```python
from build123d import *

# Parameters (mm, degrees)
SKETCH2_W                  = 25.50248159
SKETCH2_H                  = 21.40954602
BOSS_EXTRUDE1_DEPTH        = 4
M2_5_CLEARANCE_HOLE1_D     = 2.7
M2_5_CLEARANCE_HOLE1_DEPTH = 6.65
M2_5_CLEARANCE_HOLE1_TIP   = 0.811161836
SKETCH6_R                  = 4.5
CUT_EXTRUDE1_DEPTH         = 18.12268399


with BuildPart() as part:
    # Sketch2 → Boss-Extrude1 (new body)
    with BuildSketch(Plane(origin=(0, 0, 0), x_dir=(0, 0, -1), z_dir=(1, 0, 0))):
        Rectangle(SKETCH2_W, SKETCH2_H)
    extrude(amount=BOSS_EXTRUDE1_DEPTH)

    # M2.5 Clearance Hole1
    with Locations(Plane.ZY):
        with Locations((0, 7), (-6.062177826, -3.5), (6.062177826, -3.5)):
            Hole(M2_5_CLEARANCE_HOLE1_D / 2, depth=M2_5_CLEARANCE_HOLE1_DEPTH)
            with Locations((0, 0, -(M2_5_CLEARANCE_HOLE1_DEPTH + M2_5_CLEARANCE_HOLE1_TIP / 2))):  # 118° drill point
                Cone(0, M2_5_CLEARANCE_HOLE1_D / 2, M2_5_CLEARANCE_HOLE1_TIP, mode=Mode.SUBTRACT)

    # Sketch6 → Cut-Extrude1 (cut, through all)
    with BuildSketch(Plane.ZY):
        Circle(SKETCH6_R)
    extrude(amount=-CUT_EXTRUDE1_DEPTH, mode=Mode.SUBTRACT)


solid = part.part
```
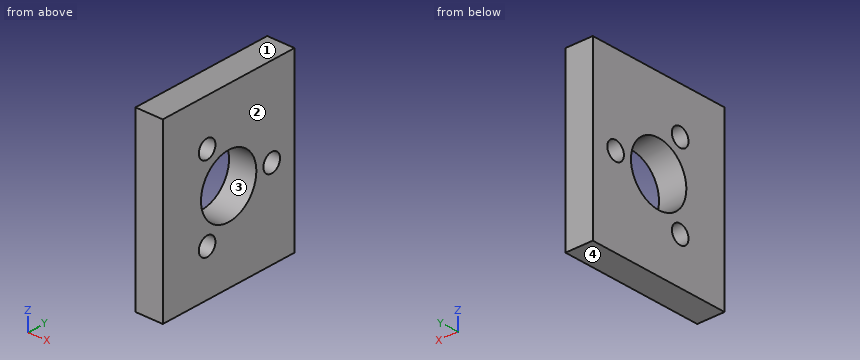
CAD build for the part. Positions are in the model's coordinates, mm. Face numbers are marked on the shaded views. Coordinates: 2 decimals unless noted, no trailing zeros. Write each loop counter-clockwise with the first axis right and the second up, starting at its lowest first coordinate (ties: lowest second). Pieces come first, ordered by that corner, then holes. Notation, with made-up numbers: (-6.5, 57.25) -> (49.5, 57.25) arc R9 ccw to (49.5, 62.25) -> close; hole circle Ø8 at (-24, 68). An arc over 180 degrees is marked (long way). Return JSON: item names as keys, results as strings. Group by question number.
Q1. Cut at C-C, the plane z = 0. Give the cut face in (x, y), then the cut area to 3 significant figures.
Q2. Cut at A-A, the plane y = 7. Give the cut face in (x, z), then the cut area to 3 significant figures.
Q3. Cut at B-B, the plane x = 0.75. Give the cut face in (y, z), then the cut area to 3 significant figures.
Q4. Pull direction Z, two halves, no side cores. Call the marked faces 1, 2, 3 and 4: released by +Z, released by -Z, zero draft, split by the parting line, or undercut.
Q5. Drill centre lines: line 1 (Y direction, x = 3.1, z = 0); line 2 (Y direction, x = 0.85, z = 0.75); line 3 (Y direction, x = 2.35, z = 6.25). Where is each one in solid material? Low to high.
Q6. Cut at D-D, the plane y = -3. Give the cut face in (x, z).
Returned:
{
 "1": {"outline": "(0, -10.7) -> (4, -10.7) -> (4, -4.5) -> (0, -4.5) -> close; (0, 4.5) -> (4, 4.5) -> (4, 5.65) -> (0, 5.65) -> close; (0, 8.35) -> (4, 8.35) -> (4, 10.7) -> (0, 10.7) -> close", "area": "38.8 mm2"},
 "2": {"outline": "(0, -12.75) -> (4, -12.75) -> (4, -1.35) -> (0, -1.35) -> close; (0, 1.35) -> (4, 1.35) -> (4, 12.75) -> (0, 12.75) -> close", "area": "91.2 mm2"},
 "3": {"outline": "(-10.7, -12.75) -> (10.7, -12.75) -> (10.7, 12.75) -> (-10.7, 12.75) -> close; hole circle Ø2.7 at (-3.5, -6.06); hole circle Ø2.7 at (-3.5, 6.06); hole circle Ø9 at (0, 0); hole circle Ø2.7 at (7, 0)", "area": "465 mm2"},
 "4": {"face 1": "released by +Z", "face 2": "zero draft", "face 3": "undercut", "face 4": "released by -Z"},
 "5": {"line 1": "y = -10.7 to -4.5, 4.5 to 5.65, 8.35 to 10.7", "line 2": "y = -10.7 to -4.44, 4.44 to 5.88, 8.12 to 10.7", "line 3": "y = -10.7 to -4.84, -2.16 to 10.7"},
 "6": {"outline": "(0, -12.75) -> (4, -12.75) -> (4, -7.32) -> (0, -7.32) -> close; (0, -4.81) -> (4, -4.81) -> (4, -3.35) -> (0, -3.35) -> close; (0, 3.35) -> (4, 3.35) -> (4, 4.81) -> (0, 4.81) -> close; (0, 7.32) -> (4, 7.32) -> (4, 12.75) -> (0, 12.75) -> close"}
}
